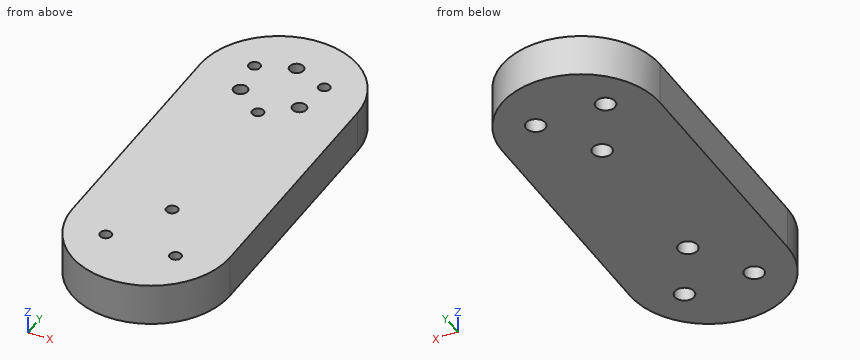
Autodesk Inventor part; units mm, degrees
ref_plane "YZ Plane" through (0, 0, 0) normal (1, 0, 0) x (0, 1, 0)
ref_plane "XZ Plane" through (0, 0, 0) normal (0, 1, 0) x (-1, 0, 0)
ref_plane "XY Plane" through (0, 0, 0) normal (0, 0, 1) x (1, 0, 0)
sketch "Sketch1" plane through (0, 0, 0) normal (0, 0, 1) x (1, 0, 0)
  circle A0 centre (0, 0) radius 22.5
  circle A1 centre (0, -70) radius 22.5
  line L0 (-22.5, 0) -> (-22.5, -70)
  line L1 (22.5, 0) -> (22.5, -70)
  circle A2 centre (0, -70) radius 11.5 construction
  circle A3 centre (0, -70) radius 9.715 construction
  line L2 (0, -20) -> (0, -150) construction
  line L3 (11.5, -70) -> (-11.5, -70) construction
  line L4 (9.9593, -64.25) -> (0, -70) construction
  line L5 (0, -70) -> (-9.9593, -64.25) construction
  line L6 (0, -70) -> (9.9593, -75.75) construction
  line L7 (0, -70) -> (-9.9593, -75.75) construction
  circle A4 centre (0, -58.5) radius 2.75
  circle A5 centre (9.9593, -75.75) radius 2.75
  circle A6 centre (-9.9593, -75.75) radius 2.75
  circle A7 centre (0, -58.5) radius 1.65
  circle A8 centre (9.9593, -75.75) radius 1.65
  circle A9 centre (-9.9593, -75.75) radius 1.65
  circle A10 centre (8.4134, -65.1425) radius 2
  circle A11 centre (0, -79.715) radius 2
  circle A12 centre (-8.4134, -65.1425) radius 2
  line L8 (-22.5, -35) -> (22.5, -35) construction
  circle A13 centre (0, 0) radius 22.5
  line L9 (9.9593, -5.75) -> (0, 0) construction
  circle A14 centre (8.4134, -4.8575) radius 2
  line L10 (0, 0) -> (9.9593, 5.75) construction
  line L11 (0, 0) -> (-9.9593, -5.75) construction
  circle A15 centre (-8.4134, -4.8575) radius 2
  circle A16 centre (0, 0) radius 9.715 construction
  circle A17 centre (0, 0) radius 11.5 construction
  circle A18 centre (0, 9.715) radius 2
  line L12 (0, 0) -> (-9.9593, 5.75) construction
  line L13 (11.5, 0) -> (-11.5, 0) construction
  circle A19 centre (-9.9593, 5.75) radius 2.75
  circle A20 centre (-9.9593, 5.75) radius 1.65
  line L14 (0, -50) -> (0, 80) construction
  circle A21 centre (0, -11.5) radius 1.65
  circle A22 centre (0, -11.5) radius 2.75
  circle A23 centre (9.9593, 5.75) radius 2.75
  circle A24 centre (9.9593, 5.75) radius 1.65
  dimension "d3" = 23
  dimension "d0" = 45
  dimension "d1" = 70
  dimension "d2" = 19.43
  dimension "d4" = 30
  dimension "d5" = 30
  dimension "d6" = 30
  dimension "d7" = 30
  dimension "d8" = 5.5
  dimension "d9" = 3.3
  dimension "d10" = 4
extrude "Extrusion1" add sketch "Sketch1" along normal blind 12 contours A0 | L1 A1 L0 A0 | A1 | A4 | A5 | A6 | A10 | A11 | A12 | A14 | A15 | A18 | A19 | A22 | A23
extrude "Extrusion2" cut sketch "Sketch1" along normal blind 5 contours A4 | A5 | A6 | A19 | A22 | A23 | A24
extrude "Extrusion3" cut sketch "Sketch1" against normal blind 5 from surface at 12 contours A14 | A15 | A18
properties part number "shank_thigh_connector"
Input: part model. Units: mm. Frame: model coordinates. Give positions to 0.01 mm unless a question says otherwise; leave off trailing zeros. Write each loop counter-clockwise with the first axis right and the second up, starting at its lowest first coordinate (ties: lowest second). Pieces come first, ordered by that corner, then holes. Notation, with made-up numbers: (78, 39.25) - (124, 39.25) arc R13 cw to (124, 44.25) - close; hole circle Ø11 at (-21, 48). An arc over 180 degrees is marked (long way). Write item = value, one per line. Start each with the question number.
1) Cut plane A-A (y = -11.5). Return loops of the section in (x, z).
2) Cut plane C-C (y = 5.75). Return loops of the section in (x, z), and give its area (3 significant figures).
3) Cut plane D-D (x = -16.5). Return loops of the section in (y, z), and give its area (3 significant figures).
4) Cut plane B-B (x = 0). Return loops of the section in (y, z) (3 decimals), and give its area (3 significant figures).
5) Material intervals for L1, parallel to Y at x = 0, z = 8.85 (3 decimals); L2, parallel to X at y = 7, z = 8; L3, parallel to Y at x = -10, z = 10.25, sorted ascending. Write a range as [from, to].
6) Pin query (flat end, axial travel): pin 1 (12 mm diameter, centred on x = 6, y = -75.5, fed in from -Z); pin 2 (3 mm diameter, centred on x = 9.96, y = -75.75, fed in from -Z); pin 3 (3 mm diameter, centred on x = -8.41, y = -4.86, fed in from +Z); pin 4 (6 mm diameter, centred on x = -8, z = 1.5, fed in from +Y). Return the tip coordinate at first contact, or that it passes through.
Answers follow:
q1.outline = (-22.5, 0) - (-2.75, 0) - (-2.75, 5) - (-1.65, 5) - (-1.65, 12) - (-22.5, 12) - close; (1.65, 5) - (2.75, 5) - (2.75, 0) - (22.5, 0) - (22.5, 12) - (1.65, 12) - close
q2.outline = (-21.75, 0) - (-12.71, 0) - (-12.71, 5) - (-11.61, 5) - (-11.61, 12) - (-21.75, 12) - close; (-8.31, 5) - (-7.21, 5) - (-7.21, 0) - (7.21, 0) - (7.21, 5) - (8.31, 5) - (8.31, 12) - (-8.31, 12) - close; (11.61, 5) - (12.71, 5) - (12.71, 0) - (21.75, 0) - (21.75, 12) - (11.61, 12) - close
q2.area = 421 mm^2
q3.outline = (-85.3, 0) - (15.3, 0) - (15.3, 12) - (-85.3, 12) - close
q3.area = 1,210 mm^2
q4.outline = (-92.5, 0) - (-61.25, 0) - (-61.25, 5) - (-60.15, 5) - (-60.15, 12) - (-92.5, 12) - close; (-56.85, 5) - (-55.75, 5) - (-55.75, 0) - (-14.25, 0) - (-14.25, 5) - (-13.15, 5) - (-13.15, 12) - (-56.85, 12) - close; (-9.85, 5) - (-8.75, 5) - (-8.75, 0) - (22.5, 0) - (22.5, 12) - (11.715, 12) - (11.715, 7) - (7.715, 7) - (7.715, 12) - (-9.85, 12) - close
q4.area = 1,260 mm^2
q5.L1 = [-92.5, -60.15], [-56.85, -13.15], [-9.85, 7.715], [11.715, 22.5]
q5.L2 = [-21.38, -11.04], [-8.88, 8.88], [11.04, 21.38]
q5.L3 = [-90.16, -77.4], [-74.1, -6.08], [-3.64, 4.1], [7.4, 20.16]
q6.pin_1 = 0
q6.pin_2 = through
q6.pin_3 = 7
q6.pin_4 = 21.94
